Verification items for the finished model (mm, model axes). Face numbers are marked on the shaded views. A direction names the side the tool comes from. Coordinates: 2 decimals unless noted, no trailing zeros. Order: outer loops, then holes, each group sorted by start corner. A loop starts at its lowest first (then second) coordinate and runs counter-clockwise, first axis right, second up. Notation, with made-up numbers: (66, 64.5) - (83, 64.5) arc R12 ccw to (83, 68.5) - close; hole circle Ø1 at (-29, 31.25). An arc over 180 degrees is marked (long way). Answer as CSV lines item,"result". Start each with the question number.
1. Section check B-B (z = 0). Record the cut outline in (x, y).
2. Material ranges on L1, parallel to Y at x = 0.55, z = 0; L2, parallel to X at y = -5.5, z = 0.5; L3, parallel to Y at x = 12.75, z = 0.25, recorded low to high. Write a range as [from, to].
3. Section check D-D (x = 16). Record the cut outline in (y, z), and give its area (3 significant figures).
4. Section check C-C (y = -23). Record the cut outline in (x, z), and give its area (3 significant figures).
5. Go/stop test with flat-tipped pins: pin 1 (6 mm diameter, centred on y = 19.5, z = -4, fed in from -X); pin 2 (4 mm diameter, centred on x = 16.5, z = -2, fed in from -Y); pin 3 (2 mm diameter, centred on y = -7.5, z = -3, fed in from +X). Record where each tip stops, or that it passes through.
6. Set-up check for the marked faces 1 and 2: record each of +Z, -Z, +X, -X, +Y, -Y from which the full face is reachable in a straight line by a thin tool's end or side.
7. Section check A-A (y = 23). Record the cut outline in (x, z).
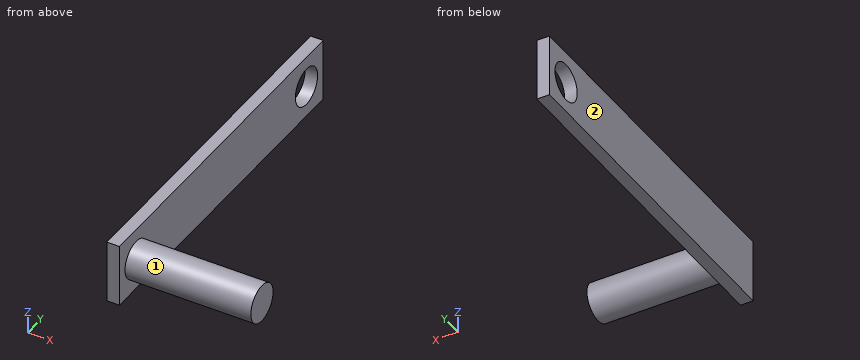
from build123d import *

# Parameters (mm, degrees)
SKETCH1_W           = 10
SKETCH1_H           = 55
BOSS_EXTRUDE1_DEPTH = 2
SKETCH2_R           = 3
CUT_EXTRUDE1_DEPTH  = 2
SKETCH3_R           = 3
BOSS_EXTRUDE2_DEPTH = 20


with BuildPart() as part:
    # Sketch1 → Boss-Extrude1 (new body)
    with BuildSketch(Plane(origin=(0, 0, 0), x_dir=(0, 0, -1), z_dir=(1, 0, 0))):
        Rectangle(SKETCH1_W, SKETCH1_H)
    extrude(amount=BOSS_EXTRUDE1_DEPTH)

    # Sketch2 → Cut-Extrude1 (cut)
    with BuildSketch(Plane(origin=(2, 0, 0), x_dir=(0, 0, -1), z_dir=(1, 0, 0))):
        with Locations((0, 23)):
            Circle(SKETCH2_R)
    extrude(amount=-CUT_EXTRUDE1_DEPTH, mode=Mode.SUBTRACT)

    # Sketch3 → Boss-Extrude2 (add)
    with BuildSketch(Plane(origin=(2, 0, 0), x_dir=(0, 0, -1), z_dir=(1, 0, 0))):
        with Locations((0, -23)):
            Circle(SKETCH3_R)
    extrude(amount=BOSS_EXTRUDE2_DEPTH)


solid = part.part
Evaluation:
1,outline,"(0, -27.5) - (2, -27.5) - (2, -26) - (22, -26) - (22, -20) - (2, -20) - (2, 20) - (0, 20) - close; (0, 26) - (2, 26) - (2, 27.5) - (0, 27.5) - close"
2,L1,"y = [-27.5, 20], [26, 27.5]"
2,L2,"x = [0, 2]"
2,L3,"y = [-25.99, -20.01]"
3,outline,"circle Ø6 at (-23, 0)"
3,area,"28.3 mm²"
4,outline,"(0, -5) - (2, -5) - (2, -3) - (22, -3) - (22, 3) - (2, 3) - (2, 5) - (0, 5) - close"
4,area,"140 mm²"
5,pin 1,"stops at x = 0"
5,pin 2,"stops at y = -26"
5,pin 3,"stops at x = 2"
6,face 1,"+X"
6,face 2,"+Z, -Z, -X, +Y, -Y"
7,outline,"(0, -5) - (2, -5) - (2, -3) - (0, -3) - close; (0, 3) - (2, 3) - (2, 5) - (0, 5) - close"
